Check sheet for the modelled part. Datum: model origin and axes. Units: mm. A direction names the side the tool comes from. Give positions to 0.01 mm unless a question says otherwise; leave off trailing zeros. Loops run counter-clockwise (first coordinate to the right, second up) from the corner with the lowest first, then second, coordinate; pieces in that order, holes last. Notation, with made-up numbers: (85, 79) -> (106, 79) arc R18 ccw to (106, 112) -> close; hole circle Ø4 at (51, 87.25). An arc over 180 degrees is marked (long way). Write each question's results on one line, items separated by ' | '. Start each with the question number.
Item 1: Access from +Z, -Z, +X, -X, +Y, -Y to the whole of each face (thin tool, end or side, straight path). Record for faces 1 (the face through (-6.084, 10.344, -5.889)), 2 (the face through (6.084, -10.344, -5.889)), 3 (the face through (5.92, 10.44, -5.89)).
Item 2: Mould release check, pull along Y, two halves, no side actions. Record for faces 4 (the face through (5.939, 11.418, -12.302)), 5 (the face through (-5.92, -10.44, -5.89)), 6 (the face through (10.77, 6.25, -0.39)), 7 (the face through (6.466, -2.681, -7.888)): pulls with the +Y half, pulls with the -Y half, needs draft (parallel to the pull), parting line crosses it, or undercut.
Item 3: Gauge pin test, flat ends, axial feed: pin 1 Ø1.5 at (x, z) = (-5, -10) entering from -Y; pin 2 Ø9.5 at (y, z) = (-1, -4.5) entering from +X; pin 3 Ø4 at (x, z) = (-8.5, -14.5) entering from +Y. Record the tip position at first contact, or that the pin passes through.
Item 4: Cross-section at A-A on z = -10.25. Enter the section's corners in (x, y).
Item 5: Scan lines: line 1 along Y through (x, z) = (0, -8.25); line 2 along X through (y, z) = (13.5, -3.75); line 3 along Y through (x, z) = (-7.5, -9.5). Record each from-to range of solid material in increasing order.
from build123d import *

# Parameters (mm, degrees)
BASENUTSKE_R   = 7
BASENUT_DEPTH  = 16
FLANGEFILLET_R = 0.96


with BuildPart() as part:
    # BaseNutSke → BaseNut (new body)
    with BuildSketch(Plane.XY):
        Polygon((12, 6.92820323), (12, -6.92820323), (0, -13.856406461), (-12, -6.92820323), (-12, 6.92820323), (0, 13.856406461), align=None)
        Circle(BASENUTSKE_R, mode=Mode.SUBTRACT)
    extrude(amount=-BASENUT_DEPTH)

    # Sketch6 → Flange (revolve)
    with BuildSketch(Plane(origin=(0, 0, 0), x_dir=(0, 0, -1), z_dir=(1, 0, 0)), mode=Mode.PRIVATE) as flange_sk:
        with BuildLine():
            Line((10.165622253, 7), (13.6, 16.435875309))
            ThreePointArc((13.6, 16.435875309), (14.977547085, 17.231202489), (16, 16.012690555))
            Line((16, 16.012690555), (16, 7))
            Line((16, 7), (10.165622253, 7))
        make_face()
    revolve(flange_sk.sketch.rotate(Axis((0, 0, 0), (0, 0, -1)), 90), axis=Axis((0, 0, 0), (0, 0, -1)))

    # Sketch3 → Double-Chamfer (revolve, cut)
    with BuildSketch(Plane(origin=(0, 0, 0), x_dir=(0, 0, -1), z_dir=(1, 0, 0)), mode=Mode.PRIVATE) as double_chamfer_sk:
        Polygon((1.6, 26.556406461), (-12.7, 26.556406461), (-12.7, 12), (0, 12), (1.6, 13.856406461), align=None)
    revolve(double_chamfer_sk.sketch.rotate(Axis((0, 0, 0), (0, 0, -1)), 90), axis=Axis((0, 0, 0), (0, 0, -1)), mode=Mode.SUBTRACT)

    # FlangeFillet
    flangefillet_edges = [part.edges().sort_by_distance(p)[0] for p in [
        (12, -3.479213152, -12.16534592),
        (12, 3.479213152, -12.16534592),
        (6, -10.392304845, -11.985473425),
        (6, 10.392304845, -11.985473425),
        (-6, 10.392304845, -11.985473425),
        (-12, 0, -11.985473425),
        (-6, -10.392304845, -11.985473425),
    ]]
    fillet(flangefillet_edges, radius=FLANGEFILLET_R)


solid = part.part
Answer sheet:
1) face 1: +Z, -X, +Y | face 2: +Z, +X, -Y | face 3: +Z, +X, +Y
2) face 4: parting line crosses it | face 5: pulls with the -Y half | face 6: pulls with the +Y half | face 7: undercut
3) pin 1: stops at y = -11.4 | pin 2: stops at x = 12 | pin 3: stops at y = 15.97
4) outline: (-12, -6.93) -> (0, -13.86) -> (12, -6.93) -> (12, 6.93) -> (0, 13.86) -> (-12, 6.93) -> close; hole circle Ø14 at (0, 0)
5) line 1: y = -13.86 to -7, 7 to 13.86 | line 2: x = -0.62 to 0.62 | line 3: y = -9.53 to 9.53
